from build123d import *

# Parameters (mm, degrees)
SKETCH_2_R          = 1.6
SKETCH_2_R_2        = 10
SKETCH_2_R_3        = 5.1
SKETCH_2_R_4        = 4
EXTRUDE_1_DEPTH     = 3
SKETCH_3_R          = 1
SKETCH_3_W          = 10
SKETCH_3_H          = 3.05
CUT_EXTRUDE_1_DEPTH = 80.507861247
FILLET_1_R          = 3


with BuildPart() as part:
    # 草图2 → 凸台-拉伸1 (new body)
    # profile 1 of 5: a face of its own
    with BuildSketch(Plane(origin=(0, 0, 0), x_dir=(0, 0, -1), z_dir=(1, 0, 0))):
        with BuildLine():
            Line((-72.5, -4), (-47.5, -4))
            Line((-47.5, -4), (-43.710028433, 3.096407942))
            ThreePointArc((-43.710028433, 3.096407942), (-40.443183901, 7.410718134), (-36, 10.5))
            Line((-36, 10.5), (-21, 10.5))
            ThreePointArc((-21, 10.5), (-18.287060326, 8.866629069), (-15.918567159, 6.764681785))
            ThreePointArc((-15.918567159, 6.764681785), (-14.470668447, 13.219829878), (-9, 9.5))
            ThreePointArc((-9, 9.5), (-9.03759069, 8.952905441), (-9.149656228, 8.416093713))
            Line((-9.149656228, 8.416093713), (-8, 12.5))
            Line((-8, 12.5), (0, 12.5))
            ThreePointArc((0, 12.5), (-10, 22.500000014), (2.8e-08, 32.5))
            ThreePointArc((2.8e-08, 32.5), (-25.937249131, 28.981693295), (-50, 18.681042995))
            Line((-50, 18.681042995), (-50, 8.681042995))
            Line((-50, 8.681042995), (-52.5, 4))
            Line((-52.5, 4), (-72.5, 4))
            Line((-72.5, 4), (-72.5, -4))
        make_face()
        with Locations((-69.5, 0)):
            Circle(SKETCH_2_R, mode=Mode.SUBTRACT)
        with Locations((-50.5, 0)):
            Circle(SKETCH_2_R, mode=Mode.SUBTRACT)
    # profile 2 of 5: a face of its own
    with BuildSketch(Plane(origin=(0, 0, 0), x_dir=(0, 0, -1), z_dir=(1, 0, 0))):
        with BuildLine():
            ThreePointArc((50, 18.681042995), (25.937249158, 28.981693288), (2.8e-08, 32.5))
            ThreePointArc((2.8e-08, 32.5), (7.071067822, 29.571067802), (10, 22.5))
            ThreePointArc((10, 22.5), (7.071067812, 15.428932188), (0, 12.5))
            Line((0, 12.5), (8, 12.5))
            Line((8, 12.5), (9.149656228, 8.416093713))
            ThreePointArc((9.149656228, 8.416093713), (12.452905441, 13.46240931), (17, 9.5))
            ThreePointArc((17, 9.5), (16.719829878, 8.029331553), (15.918567159, 6.764681785))
            ThreePointArc((15.918567159, 6.764681785), (18.287060326, 8.866629069), (21, 10.5))
            Line((21, 10.5), (36, 10.5))
            ThreePointArc((36, 10.5), (40.443183901, 7.410718134), (43.710028433, 3.096407942))
            Line((43.710028433, 3.096407942), (47.5, -4))
            Line((47.5, -4), (72.5, -4))
            Line((72.5, -4), (72.5, 4))
            Line((72.5, 4), (52.5, 4))
            Line((52.5, 4), (50, 8.681042995))
            Line((50, 8.681042995), (50, 18.681042995))
        make_face()
        with Locations((50.5, 0)):
            Circle(SKETCH_2_R, mode=Mode.SUBTRACT)
        with Locations((69.5, 0)):
            Circle(SKETCH_2_R, mode=Mode.SUBTRACT)
    # profile 3 of 5: a face of its own
    with BuildSketch(Plane(origin=(0, 0, 0), x_dir=(0, 0, -1), z_dir=(1, 0, 0))):
        with Locations((0, 22.5)):
            Circle(SKETCH_2_R_2)
        with Locations((0, 22.5)):
            Circle(SKETCH_2_R_3, mode=Mode.SUBTRACT)
    # profile 4 of 5: a face of its own
    with BuildSketch(Plane(origin=(0, 0, 0), x_dir=(0, 0, -1), z_dir=(1, 0, 0))):
        with Locations((-13, 9.5)):
            Circle(SKETCH_2_R_4)
        with Locations((-13, 9.5)):
            Circle(SKETCH_2_R, mode=Mode.SUBTRACT)
    # profile 5 of 5: a face of its own
    with BuildSketch(Plane(origin=(0, 0, 0), x_dir=(0, 0, -1), z_dir=(1, 0, 0))):
        with Locations((13, 9.5)):
            Circle(SKETCH_2_R_4)
        with Locations((13, 9.5)):
            Circle(SKETCH_2_R, mode=Mode.SUBTRACT)
    extrude(amount=EXTRUDE_1_DEPTH)

    # 草图3 → 切除-拉伸1 (cut, through all)
    with BuildSketch(Plane(origin=(3, 0, 0), x_dir=(0, 0, -1), z_dir=(1, 0, 0))):
        with Locations((-43, 16.525)):
            Circle(SKETCH_3_R)
        with Locations((-43, 13.475)):
            Circle(SKETCH_3_R)
        with Locations((-35, 16.525)):
            Circle(SKETCH_3_R)
        with Locations((-35, 13.475)):
            Circle(SKETCH_3_R)
        with Locations((-25, 16.525)):
            Circle(SKETCH_3_R)
        with Locations((-17, 16.525)):
            Circle(SKETCH_3_R)
        with Locations((-17, 13.475)):
            Circle(SKETCH_3_R)
        with Locations((-25, 13.475)):
            Circle(SKETCH_3_R)
        with Locations((25, 13.475)):
            Circle(SKETCH_3_R)
        with Locations((17, 13.475)):
            Circle(SKETCH_3_R)
        with Locations((17, 16.525)):
            Circle(SKETCH_3_R)
        with Locations((25, 16.525)):
            Circle(SKETCH_3_R)
        with Locations((35, 13.475)):
            Circle(SKETCH_3_R)
        with Locations((35, 16.525)):
            Circle(SKETCH_3_R)
        with Locations((43, 13.475)):
            Circle(SKETCH_3_R)
        with Locations((43, 16.525)):
            Circle(SKETCH_3_R)
        with Locations((-21, 15)):
            Rectangle(SKETCH_3_W, SKETCH_3_H)
        with Locations((-39, 15)):
            Rectangle(SKETCH_3_W, SKETCH_3_H)
        with Locations((21, 15)):
            Rectangle(SKETCH_3_W, SKETCH_3_H)
        with Locations((39, 15)):
            Rectangle(SKETCH_3_W, SKETCH_3_H)
    extrude(amount=-CUT_EXTRUDE_1_DEPTH, mode=Mode.SUBTRACT)

    # 圆角1
    fillet_1_edges = [part.edges().sort_by_distance(p)[0] for p in [
        (1.5, 10.5, 36),
        (1.5, -4, 47.5),
        (1.5, 4, 52.5),
        (1.5, 8.681042995, 50),
        (1.5, 18.681042995, 50),
        (1.5, 18.681042995, -50),
        (1.5, 8.681042995, -50),
        (1.5, 4, -52.5),
        (1.5, -4, -47.5),
        (1.5, 10.5, -36),
        (1.5, 10.5, -21),
        (1.5, 12.5, -8),
        (1.5, 12.5, 8),
        (1.5, 10.5, 21),
    ]]
    fillet(fillet_1_edges, radius=FILLET_1_R)


solid = part.part
Work out the finished part from the listing and answer in its coordinate system (mm). A direction names the side the tool comes from. Give positions to 0.01 mm unless a question says otherwise; leave off trailing zeros. Write each loop counter-clockwise with the first axis right and the second up, starting at its lowest first coordinate (ties: lowest second). Pieces come first, ordered by that corner, then holes. Notation, with made-up numbers: M 37,21.25 L 75,21.25 A23 cw 75,47.25 Z; hole C 49.5,22.5 d8. An arc over 180 degrees is marked long. Answer as CSV lines item,"result".
Q1. The mould has two halves that part along Z. Classify faces 1 (the flat face through (2, 16.525, 21)), 2 (the flat face through (1, 0, -72.5)), 3 (the flat face through (1, -4, 61)): +Z half, -Z half, draft (parallel to the pull), parting line (faces both ways), or undercut.
A:
face 1,"undercut"
face 2,"-Z half"
face 3,"draft"
Q2. Given P1, Ø0.9, axis at x = 1.5, z = 65.5, coming from the +Y side; P2, Ø1, axis at x = 0.5, y = 24.5, coming from the +Z side; P3, Ø1, axis at x = 2, y = 8, coming from the -Z side; P4, Ø12, axis at y = 2, z = 31, coming from the -X side, each flat-ended and moving along its own axis, determine where each tip first touches the part or whether it passes through.
A:
P1,"stops at y = 4"
P2,"stops at z = 39.79"
P3,"stops at z = -50.63"
P4,"passes through"
Q3. A tool of negligible diameter and unlimited length cuts with its end or side. For faces 4 (the cylindrical face through (1.521, 11.908, 7.517)), 5 (the flat face through (2, 15, 34)), 6 (the flat face through (1, 4, -64)), from which of +Z, -Z, +X, -X, +Y, -Y can it reach the whole face along a straight path? Write none if from no direction.
A:
face 4,"+X, -X, -Y"
face 5,"+X, -X"
face 6,"-Z, +X, -X, +Y"
Q4. A cutting plane is placed at C-C on x = 1.05. Count the separate pieces of the cut face and the enclosed holes in it, plus the area to 3 significant figures.
A:
separate pieces,"1"
enclosed holes,"11"
area,"2,090 mm²"
Q5. A cutting plane is placed at A-A on z = -69.5. Write down the section's boundary in (x, y).
A:
outline,"M 0,-4 L 3,-4 L 3,-1.6 L 0,-1.6 Z; M 0,1.6 L 3,1.6 L 3,4 L 0,4 Z"
Q6. A cutting plane is placed at D-D on y = 24. Write down the section's boundary in (x, z).
A:
outline,"M 0,-39.79 L 3,-39.79 L 3,-4.87 L 0,-4.87 Z; M 0,4.87 L 3,4.87 L 3,39.79 L 0,39.79 Z"
Q7. Find the intervals of material crossed by probe 1 along Y at (x, z) = (1.7, 0); probe 2 along Y at (x, z) = (1, 69.5); probe 3 along Z at (x, y) = (1.6, -2), in increasing order. Write a range as [from, to].
A:
probe 1,"y = [12.5, 17.4], [27.6, 32.5]"
probe 2,"y = [-4, -1.6], [1.6, 4]"
probe 3,"z = [-72.5, -46.43], [46.43, 72.5]"
Q8. A cutting plane is placed at B-B on y = 0. Write down the section's boundary in (x, z).
A:
outline,"M 0,-72.5 L 3,-72.5 L 3,-71.1 L 0,-71.1 Z; M 0,-67.9 L 3,-67.9 L 3,-52.1 L 0,-52.1 Z; M 0,-48.9 L 3,-48.9 L 3,-45.36 L 0,-45.36 Z; M 0,45.36 L 3,45.36 L 3,48.9 L 0,48.9 Z; M 0,52.1 L 3,52.1 L 3,67.9 L 0,67.9 Z; M 0,71.1 L 3,71.1 L 3,72.5 L 0,72.5 Z"
